from build123d import *

# Parameters (mm, degrees)
BOSS_EXTRUDE1_DEPTH      = 5
BOSS_EXTRUDE1_DEPTH_BACK = 5
SKETCH1_R                = 1.76
SKETCH1_R_2              = 2.5
CUT_EXTRUDE1_DEPTH       = 3
CUT_EXTRUDE1_DEPTH_BACK  = 3
SKETCH1_4_R              = 2.5
FILLET1_R                = 2


with BuildPart() as part:
    # Sketch1 → Boss-Extrude1 (new, two sides: drawn at the far end of the back side and taken through both)
    # profile 1 of 2: a face of its own
    with BuildSketch(Plane.XY.offset(-BOSS_EXTRUDE1_DEPTH_BACK)):
        with BuildLine():
            Line((-7.967960843, 2.96), (-27.589132312, 2.96))
            ThreePointArc((-27.589132312, 2.96), (-30.549132312, 0), (-27.589132312, -2.96))
            Line((-27.589132312, -2.96), (-7.967960843, -2.96))
            ThreePointArc((-7.967960843, -2.96), (-8.5, 0), (-7.967960843, 2.96))
        make_face()
        with Locations((-27.589132312, 0)):
            Circle(SKETCH1_R, mode=Mode.SUBTRACT)
    # profile 2 of 2: a face of its own
    with BuildSketch(Plane.XY.offset(-BOSS_EXTRUDE1_DEPTH_BACK)):
        with BuildLine():
            Line((-5.589132312, 2.96), (-7.967960843, 2.96))
            ThreePointArc((-7.967960843, 2.96), (-8.5, 0), (-7.967960843, -2.96))
            Line((-7.967960843, -2.96), (-5.589132312, -2.96))
            Line((-5.589132312, -2.96), (-4.142219081, -4.340739694))
            ThreePointArc((-4.142219081, -4.340739694), (6, 0), (-4.142219081, 4.340739694))
            Line((-4.142219081, 4.340739694), (-5.589132312, 2.96))
        make_face()
        Circle(SKETCH1_R_2, mode=Mode.SUBTRACT)
    extrude(amount=BOSS_EXTRUDE1_DEPTH + BOSS_EXTRUDE1_DEPTH_BACK)

    # Sketch1_4 → Cut-Extrude1 (cut, two sides: drawn at the far end of the back side and taken through both)
    # profile 1 of 2: a face of its own
    with BuildSketch(Plane.XY.offset(-CUT_EXTRUDE1_DEPTH_BACK)):
        with BuildLine():
            ThreePointArc((8.5, 0), (1.503717532, 8.365932918), (-7.967960843, 2.96))
            Line((-7.967960843, 2.96), (-5.589132312, 2.96))
            Line((-5.589132312, 2.96), (-4.142219081, 4.340739694))
            ThreePointArc((-4.142219081, 4.340739694), (6, 0), (-4.142219081, -4.340739694))
            Line((-4.142219081, -4.340739694), (-5.589132312, -2.96))
            Line((-5.589132312, -2.96), (-7.967960843, -2.96))
            ThreePointArc((-7.967960843, -2.96), (1.503717532, -8.365932918), (8.5, 0))
        make_face()
    # profile 2 of 2: a face of its own
    with BuildSketch(Plane.XY.offset(-CUT_EXTRUDE1_DEPTH_BACK)):
        with BuildLine():
            Line((-5.589132312, 2.96), (-7.967960843, 2.96))
            ThreePointArc((-7.967960843, 2.96), (-8.5, 0), (-7.967960843, -2.96))
            Line((-7.967960843, -2.96), (-5.589132312, -2.96))
            Line((-5.589132312, -2.96), (-4.142219081, -4.340739694))
            ThreePointArc((-4.142219081, -4.340739694), (6, 0), (-4.142219081, 4.340739694))
            Line((-4.142219081, 4.340739694), (-5.589132312, 2.96))
        make_face()
        Circle(SKETCH1_4_R, mode=Mode.SUBTRACT)
    extrude(amount=CUT_EXTRUDE1_DEPTH + CUT_EXTRUDE1_DEPTH_BACK, mode=Mode.SUBTRACT)

    # Fillet1
    fillet1_edges = [part.edges().sort_by_distance(p)[0] for p in [
        (-7.967960843, -2.96, 0),
        (-7.967960843, 2.96, 0),
    ]]
    fillet(fillet1_edges, radius=FILLET1_R)


solid = part.part
Here's how the part is built. I have some questions about the finished solid (model axes, mm). A direction names the side the tool comes from. Round coordinates to 2 decimals unless told otherwise and drop trailing zeros. Loops run counter-clockwise (first coordinate to the right, second up) from the corner with the lowest first, then second, coordinate; pieces in that order, holes last. Notation, with made-up numbers: (66.25, 73) -> (124.25, 73) arc R21 ccw to (124.25, 107) -> close; hole circle Ø9 at (80, 21.25). An arc over 180 degrees is marked (long way). Write each question's results on one line, items separated by ' | '.
(1) If we section it at D-D, the plane y = -4: List the corners of the cut face in (x, z) for me.
Worked answers:
outline: (-4.5, -5) -> (4.47, -5) -> (4.47, -3) -> (-4.5, -3) -> close; (-4.5, 3) -> (4.47, 3) -> (4.47, 5) -> (-4.5, 5) -> close
(2) If we section it at C-C, the plane z = -4.5: List the corners of the cut face in (x, y) for me.
Worked answers:
outline: (-27.59, -2.96) -> (-5.59, -2.96) -> (-4.14, -4.34) arc R6 ccw (long way) to (-4.14, 4.34) -> (-5.59, 2.96) -> (-27.59, 2.96) arc R2.96 ccw to start; hole circle Ø3.52 at (-27.59, 0); hole circle Ø5 at (0, 0)
(3) We'd pull the mould along X, two halves only. Please class faces 1 (the face through (-4.856, 3.66, -4.014)), 2 (the face through (6, 0, -4)), 3 (the face through (-0.54, -2.44, -4.01)), 4 (the face through (-8.994, 2.325, 0.042)): released by +X, released by -X, zero draft, split by the parting line, or undercut.
Worked answers:
face 1: released by -X | face 2: split by the parting line | face 3: undercut | face 4: released by +X
(4) If I drill on L1, parallel to Y at x = 0, z = -4.35; L2, parallel to Z at x = -9, y = -2.75; L3, parallel to X at y = 0.5, z = -2, over which ranges is the centre line in solid material (lowest first)?
Worked answers:
L1: -6 to -2.5, 2.5 to 6 | L2: -5 to -3, 3 to 5 | L3: -30.51 to -29.28, -25.9 to -8.49
(5) If we section it at A-A, the plane y = 0: List the corners of the cut face in (x, z) for me.
Worked answers:
outline: (-30.55, -5) -> (-29.35, -5) -> (-29.35, 5) -> (-30.55, 5) -> close; (-25.83, -5) -> (-2.5, -5) -> (-2.5, -3) -> (-8.5, -3) -> (-8.5, 3) -> (-2.5, 3) -> (-2.5, 5) -> (-25.83, 5) -> close; (2.5, -5) -> (6, -5) -> (6, -3) -> (2.5, -3) -> close; (2.5, 3) -> (6, 3) -> (6, 5) -> (2.5, 5) -> close
(6) For P1, Ø3, axis at x = -14, z = -2.5, coming from the +Y side; P2, Ø1.5, axis at x = -13, y = 3, coming from the -Z side; P3, Ø3, axis at y = -3.5, z = 3, coming from the -X side, each with a flat end and sliding along its axis, tell me the tip position at first contact or that it passes through.
Worked answers:
P1: y = 2.96 | P2: z = -5 | P3: x = -29.77
(7) If we section it at B-B, the plane x = 0: List the corners of the cut face in (y, z) for me, then the cut area to 3 significant figures.
Worked answers:
outline: (-6, -5) -> (-2.5, -5) -> (-2.5, -3) -> (-6, -3) -> close; (-6, 3) -> (-2.5, 3) -> (-2.5, 5) -> (-6, 5) -> close; (2.5, -5) -> (6, -5) -> (6, -3) -> (2.5, -3) -> close; (2.5, 3) -> (6, 3) -> (6, 5) -> (2.5, 5) -> close | area: 28.0 mm2
(8) For faces 5 (the face through (-17, -2.96, 0)), 6 (the face through (-8.5, 0, 0)), 7 (the face through (-16, 2.96, 0)), which set-ups out of +Z, -Z, +X, -X, +Y, -Y let a thin tool reach every point of the face, with its end or its side?
Worked answers:
face 5: +Z, -Z, -X, -Y | face 6: +X | face 7: +Z, -Z, -X, +Y
